Can you work these out from the model? Positions are in its coordinate system, mm. A direction names the side the tool comes from. Give positions to 0.01 mm unless a question says otherwise; leave off trailing zeros. Order: outer loops, then holes, each group sorted by start corner. A loop starts at its lowest first (then second) coordinate and runs counter-clockwise, first axis right, second up.
```python
from build123d import *

# Parameters (mm, degrees)
SKETCH_1_R               = 37.5
SKETCH_1_R_2             = 2.75
EXTRUDE_1_DEPTH          = 20
SKETCH_2_R               = 22.536189363
CUT_EXTRUDE_1_DEPTH      = 12
SKETCH_8_R               = 37.5
SKETCH_8_R_2             = 27.240226037
CUT_EXTRUDE_4_DEPTH      = 10
SKETCH_9_R               = 8
CUT_EXTRUDE_5_DEPTH      = 10
EXTRUDE_2_DEPTH          = 10
SKETCH_11_R              = 45
EXTRUDE_3_DEPTH          = 5
SKETCH_13_R              = 1.5
CUT_EXTRUDE_6_DEPTH      = 10
SKETCH_14_R              = 22.536189363
CUT_EXTRUDE_7_DEPTH      = 24
SKETCH_15_W              = 20
SKETCH_15_H              = 12
CUT_EXTRUDE_8_DEPTH      = 46
CUT_EXTRUDE_8_DEPTH_BACK = 46
SKETCH_17_R              = 45
CUT_EXTRUDE_11_DEPTH     = 10
SKETCH_19_R              = 22.536189363
EXTRUDE_4_DEPTH          = 2.5
EXTRUDE_4_DEPTH_BACK     = 2.5
SKETCH_21_R              = 1.5
CUT_EXTRUDE_12_DEPTH     = 33.5
SKETCH_22_R              = 22.536189363
EXTRUDE_6_DEPTH          = 2.5


with BuildPart() as part:
    # 草图1 → 凸台-拉伸1 (new body)
    with BuildSketch(Plane.XY):
        Circle(SKETCH_1_R)
        with Locations((-27, 16)):
            Circle(SKETCH_1_R_2, mode=Mode.SUBTRACT)
        with Locations((27, 16)):
            Circle(SKETCH_1_R_2, mode=Mode.SUBTRACT)
        with Locations((-27, -16)):
            Circle(SKETCH_1_R_2, mode=Mode.SUBTRACT)
        with Locations((27, -16)):
            Circle(SKETCH_1_R_2, mode=Mode.SUBTRACT)
    extrude(amount=EXTRUDE_1_DEPTH)

    # 草图2 → 切除-拉伸1 (cut)
    with BuildSketch(Plane.XY.offset(20)):
        Circle(SKETCH_2_R)
    extrude(amount=-CUT_EXTRUDE_1_DEPTH, mode=Mode.SUBTRACT)

    # 草图8 → 切除-拉伸4 (cut)
    with BuildSketch(Plane(origin=(0, 0, 0), x_dir=(-1, 0, 0), z_dir=(0, 0, -1))):
        Circle(SKETCH_8_R)
        Circle(SKETCH_8_R_2, mode=Mode.SUBTRACT)
    extrude(amount=-CUT_EXTRUDE_4_DEPTH, mode=Mode.SUBTRACT)

    # 草图9 → 切除-拉伸5 (cut)
    with BuildSketch(Plane(origin=(0, 0, 0), x_dir=(-1, 0, 0), z_dir=(0, 0, -1))):
        with Locations((-27, 16)):
            Circle(SKETCH_9_R)
        with Locations((27, 16)):
            Circle(SKETCH_9_R)
        with Locations((-27, -16)):
            Circle(SKETCH_9_R)
        with Locations((27, -16)):
            Circle(SKETCH_9_R)
    extrude(amount=-CUT_EXTRUDE_5_DEPTH, mode=Mode.SUBTRACT)

    # 草图10 → 凸台-拉伸2 (add)
    with BuildSketch(Plane(origin=(0, 0, 0), x_dir=(-1, 0, 0), z_dir=(0, 0, -1))):
        with BuildLine():
            ThreePointArc((-19.565154934, -18.95348588), (0, -27.240226037), (19.565154934, -18.95348588))
            ThreePointArc((19.565154934, -18.95348588), (20.117667731, -11.921580878), (26.020436633, -8.060198012))
            ThreePointArc((26.020436633, -8.060198012), (27.240226037, 0), (26.020436633, 8.060198012))
            ThreePointArc((26.020436633, 8.060198012), (20.117667731, 11.921580878), (19.565154934, 18.95348588))
            ThreePointArc((19.565154934, 18.95348588), (0, 27.240226037), (-19.565154934, 18.95348588))
            ThreePointArc((-19.565154934, 18.95348588), (-20.117667731, 11.921580878), (-26.020436633, 8.060198012))
            ThreePointArc((-26.020436633, 8.060198012), (-27.240226037, 0), (-26.020436633, -8.060198012))
            ThreePointArc((-26.020436633, -8.060198012), (-20.117667731, -11.921580878), (-19.565154934, -18.95348588))
        make_face()
    extrude(amount=EXTRUDE_2_DEPTH)

    # 草图11 → 凸台-拉伸3 (add)
    with BuildSketch(Plane(origin=(0, 0, -10), x_dir=(-1, 0, 0), z_dir=(0, 0, -1))):
        Circle(SKETCH_11_R)
    extrude(amount=EXTRUDE_3_DEPTH)

    # 草图13 → 切除-拉伸6 (cut)
    with BuildSketch(Plane(origin=(0, 0, -15), x_dir=(-1, 0, 0), z_dir=(0, 0, -1))):
        with Locations((0, 36.415999231)):
            Circle(SKETCH_13_R)
        with Locations((-36.415999231, 0)):
            Circle(SKETCH_13_R)
        with Locations((0, -36.415999231)):
            Circle(SKETCH_13_R)
        with Locations((36.415999231, 0)):
            Circle(SKETCH_13_R)
    extrude(amount=-CUT_EXTRUDE_6_DEPTH, mode=Mode.SUBTRACT)

    # 草图14 → 切除-拉伸7 (cut, through all)
    with BuildSketch(Plane.XY.offset(8)):
        Circle(SKETCH_14_R)
    extrude(amount=-CUT_EXTRUDE_7_DEPTH, mode=Mode.SUBTRACT)

    # 草图15 → 切除-拉伸8 (cut, two sides)
    with BuildSketch(Plane(origin=(0, 0, 0), x_dir=(1, 0, 0), z_dir=(0, 1, 0))) as cut_extrude_8_sk:
        Rectangle(SKETCH_15_W, SKETCH_15_H)
    extrude(amount=CUT_EXTRUDE_8_DEPTH, mode=Mode.SUBTRACT)
    extrude(cut_extrude_8_sk.sketch, amount=-CUT_EXTRUDE_8_DEPTH_BACK, mode=Mode.SUBTRACT)

    # 草图17 → 切除-拉伸11 (cut)
    with BuildSketch(Plane.XY.offset(-10)):
        Circle(SKETCH_17_R)
    extrude(amount=-CUT_EXTRUDE_11_DEPTH, mode=Mode.SUBTRACT)

    # 草图19 → 凸台-拉伸4 (add, two sides)
    with BuildSketch(Plane(origin=(0, 0, -10), x_dir=(-1, 0, 0), z_dir=(0, 0, -1))) as extrude_4_sk:
        Circle(SKETCH_19_R)
    extrude(amount=EXTRUDE_4_DEPTH)
    extrude(extrude_4_sk.sketch, amount=-EXTRUDE_4_DEPTH_BACK)

    # 草图21 → 切除-拉伸12 (cut, through all)
    with BuildSketch(Plane(origin=(0, 0, -12.5), x_dir=(-1, 0, 0), z_dir=(0, 0, -1))):
        with Locations((0, 7)):
            Circle(SKETCH_21_R)
        with Locations((-7, 0)):
            Circle(SKETCH_21_R)
        with Locations((7, 0)):
            Circle(SKETCH_21_R)
        with Locations((0, -7)):
            Circle(SKETCH_21_R)
    extrude(amount=-CUT_EXTRUDE_12_DEPTH, mode=Mode.SUBTRACT)

    # 草图22 → 凸台-拉伸6 (add)
    with BuildSketch(Plane(origin=(0, 0, -10), x_dir=(-1, 0, 0), z_dir=(0, 0, -1))):
        with BuildLine():
            ThreePointArc((-26.020436633, 8.060198012), (-27.240226037, 0), (-26.020436633, -8.060198012))
            ThreePointArc((-26.020436633, -8.060198012), (-20.117667731, -11.921580878), (-19.565154934, -18.95348588))
            ThreePointArc((-19.565154934, -18.95348588), (0, -27.240226037), (19.565154934, -18.95348588))
            ThreePointArc((19.565154934, -18.95348588), (20.117667731, -11.921580878), (26.020436633, -8.060198012))
            ThreePointArc((26.020436633, -8.060198012), (27.240226037, 0), (26.020436633, 8.060198012))
            ThreePointArc((26.020436633, 8.060198012), (20.117667731, 11.921580878), (19.565154934, 18.95348588))
            ThreePointArc((19.565154934, 18.95348588), (0, 27.240226037), (-19.565154934, 18.95348588))
            ThreePointArc((-19.565154934, 18.95348588), (-20.117667731, 11.921580878), (-26.020436633, 8.060198012))
        make_face()
        Circle(SKETCH_22_R, mode=Mode.SUBTRACT)
    extrude(amount=EXTRUDE_6_DEPTH)


solid = part.part
```
1) If I drill on line 1 (Y direction, x = -27, z = 16); line 2 (X direction, y = 16, z = 16); line 3 (Z direction, x = 19, y = -26.5), over which ranges is the centre line in solid material (lowest first)?
2) Suppose I cut it at A-A (z = 3). Please give me the cut outline in (x, y).
3) I'm going to push flat-ended pins straight in: pin 1 Ø5 at (x, y) = (7, 0) entering from +Z; pin 2 Ø2.5 at (x, y) = (0, -7) entering from +Z; pin 3 Ø7 at (x, y) = (27, -16) entering from -Z; pin 4 Ø8 at (x, z) = (-16, 2.5) entering from +Y. Where does each tip first touch, or does it pass through?
4) Suppose I cut it at D-D (y = 23.5). Please give me the cut outline in (x, z).
5) Suppose I cut it at C-C (x = 0). Please give me the cut outline in (y, z), and give its area (3 significant figures).
6) Which directions (+Z, -Z, +X, -X, +Y, -Y) give clear straight access to the entire face, cutting with the end or side of a thin tool? Please do faces 1 (the face through (-29.747, -15.879, 14.93)), 2 (the face through (0, -24, -6)), 3 (the face through (20, -14, 10)), 4 (the face through (21.496, 6.769, 6.443)).
7) Suppose I cut it at B-B (y = 0). Please give me the cut outline in (x, z).
8) We'd pull the mould along Y, two halves only. Please class faces 5 (the face through (-4.88, 37.18, 14.93)), 6 (the face through (-10, 23, 0)), 7 (the face through (-29.747, 16.121, 14.93)): +Y half, -Y half, draft (parallel to the pull), parting line (faces both ways), or undercut.
Results:
1. line 1: y = -26.02 to -18.75, -13.25 to 13.25, 18.75 to 26.02
1. line 2: x = -33.92 to -29.75, -24.25 to -15.87, 15.87 to 24.25, 29.75 to 33.92
1. line 3: z = 10 to 20
2. outline: (-26.02, -8.06) arc R8 cw to (-19.57, -18.95) arc R27.24 ccw to (-10, -25.34) - (-10, -20.2) arc R22.54 cw to (-10, 20.2) - (-10, 25.34) arc R27.24 ccw to (-19.57, 18.95) arc R8 cw to (-26.02, 8.06) arc R27.24 ccw to start; (10, -25.34) arc R27.24 ccw to (19.57, -18.95) arc R8 cw to (26.02, -8.06) arc R27.24 ccw to (26.02, 8.06) arc R8 cw to (19.57, 18.95) arc R27.24 ccw to (10, 25.34) - (10, 20.2) arc R22.54 cw to (10, -20.2) - close
3. pin 1: stops at z = -7.5
3. pin 2: passes through
3. pin 3: stops at z = 10
3. pin 4: stops at y = 24.45
4. outline: (-29.22, 10) - (-13.78, 10) - (-13.78, -12.5) - (13.78, -12.5) - (13.78, 10) - (29.22, 10) - (29.22, 20) - (-29.22, 20) - close; hole (-10, -6) - (10, -6) - (10, 6) - (-10, 6) - close
5. outline: (-37.5, 10) - (-27.24, 10) - (-27.24, 6) - (-22.54, 6) - (-22.54, 20) - (-37.5, 20) - close; (-27.24, -12.5) - (-8.5, -12.5) - (-8.5, -7.5) - (-22.54, -7.5) - (-22.54, -6) - (-27.24, -6) - close; (-5.5, -12.5) - (5.5, -12.5) - (5.5, -7.5) - (-5.5, -7.5) - close; (8.5, -12.5) - (27.24, -12.5) - (27.24, -6) - (22.54, -6) - (22.54, -7.5) - (8.5, -7.5) - close; (22.54, 6) - (27.24, 6) - (27.24, 10) - (37.5, 10) - (37.5, 20) - (22.54, 20) - close
5. area: 593 mm2
6. face 1: +Z, -Z
6. face 2: +Y, -Y
6. face 3: -Z
6. face 4: +Z
7. outline: (-37.5, 10) - (-27.24, 10) - (-27.24, -12.5) - (-8.5, -12.5) - (-8.5, -7.5) - (-22.54, -7.5) - (-22.54, 20) - (-37.5, 20) - close; (-5.5, -12.5) - (5.5, -12.5) - (5.5, -7.5) - (-5.5, -7.5) - close; (8.5, -12.5) - (27.24, -12.5) - (27.24, 10) - (37.5, 10) - (37.5, 20) - (22.54, 20) - (22.54, -7.5) - (8.5, -7.5) - close
8. face 5: parting line
8. face 6: draft
8. face 7: undercut
